from build123d import *

# Parameters (mm, degrees)
SKETCH_1_R          = 29.5
EXTRUDE_1_DEPTH     = 6.6
SKETCH_2_R          = 2
CUT_EXTRUDE_1_DEPTH = 6.6
SKETCH_3_R          = 4
CUT_EXTRUDE_2_DEPTH = 6.6


with BuildPart() as part:
    # 草图1 → 凸台-拉伸1 (new body)
    with BuildSketch(Plane(origin=(0, 0, 0), x_dir=(0, 0, -1), z_dir=(1, 0, 0))):
        Circle(SKETCH_1_R)
    extrude(amount=EXTRUDE_1_DEPTH)

    # 草图2 → 切除-拉伸1 (cut)
    with BuildSketch(Plane(origin=(6.6, 0, 0), x_dir=(0, 0, -1), z_dir=(1, 0, 0))):
        with Locations((0, 17.25)):
            Circle(SKETCH_2_R)
        with Locations((14.938938215, 8.625)):
            Circle(SKETCH_2_R)
        with Locations((14.938938215, -8.625)):
            Circle(SKETCH_2_R)
        with Locations((0, -17.25)):
            Circle(SKETCH_2_R)
        with Locations((-14.938938215, -8.625)):
            Circle(SKETCH_2_R)
        with Locations((-14.938938215, 8.625)):
            Circle(SKETCH_2_R)
    extrude(amount=-CUT_EXTRUDE_1_DEPTH, mode=Mode.SUBTRACT)

    # 草图3 → 切除-拉伸2 (cut)
    with BuildSketch(Plane(origin=(6.6, 0, 0), x_dir=(0, 0, -1), z_dir=(1, 0, 0))):
        Circle(SKETCH_3_R)
    extrude(amount=-CUT_EXTRUDE_2_DEPTH, mode=Mode.SUBTRACT)


solid = part.part
Source: CAD feature listing. Evaluate the final solid. Frame: model axes, mm. Round coordinates to 2 decimals unless told otherwise and drop trailing zeros. Write each loop counter-clockwise with the first axis right and the second up, starting at its lowest first coordinate (ties: lowest second). Pieces come first, ordered by that corner, then holes. Notation, with made-up numbers: M -1,-33 L 3,-33 A14 cw 3,-13 Z; hole C -13,5 d4. An arc over 180 degrees is marked long. One line per item, written item: value. Start each with the question number.
Item 1: Section query C-C (y = -9.5). Return the cut outline in (x, z).
Item 2: Section query A-A (y = 0). Return the cut outline in (x, z).
Item 3: Ray query, L1, parallel to Z at x = 3, y = -7.5; L2, parallel to Z at x = 2.25, y = 8; L3, parallel to Z at x = 4.75, y = -16.5. Return the intervals inside material, ascending. Write a range as from..to.
Item 4: Section query B-B (z = 0). Return the cut outline in (x, y).
Item 5: Pin query (flat end, axial travel): pin 1 (1.5 mm diameter, centred on x = 2, z = -8.5, fed in from +Y); pin 2 (3 mm diameter, centred on y = 17.25, z = 0, fed in from -X); pin 3 (1 mm diameter, centred on x = 4, z = -10, fed in from +Y); pin 4 (3 mm diameter, centred on x = 0.5, z = -8, fed in from +Y) (3 decimals). Return the tip coordinate at first contact, or that it passes through.
Item 6: Section query D-D (x = 3). Return the cut outline in (y, z) (3 decimals), plus the area to 3 significant figures.
Item 7: Mould query, pull axis Y, two halves, no side actions, for faces 1 (the cylindrical face through (3.25, 8.86, -28.14)), 2 (the flat face through (0, -6, 0)), 3 (the cylindrical face through (3.35, 8.71, -12.94)). Classes: pulls with the +Y half, pulls with the -Y half, needs draft (parallel to the pull), parting line crosses it, or undercut.
Result set:
1. outline: M 0,-27.93 L 6.6,-27.93 L 6.6,-16.74 L 0,-16.74 Z; M 0,-13.14 L 6.6,-13.14 L 6.6,13.14 L 0,13.14 Z; M 0,16.74 L 6.6,16.74 L 6.6,27.93 L 0,27.93 Z
2. outline: M 0,-29.5 L 6.6,-29.5 L 6.6,-4 L 0,-4 Z; M 0,4 L 6.6,4 L 6.6,29.5 L 0,29.5 Z
3. L1: z = -28.53..-16.59, -13.29..13.29, 16.59..28.53
3. L2: z = -28.39..-16.84, -13.04..13.04, 16.84..28.39
3. L3: z = -24.45..-1.85, 1.85..24.45
4. outline: M 0,-29.5 L 6.6,-29.5 L 6.6,-19.25 L 0,-19.25 Z; M 0,-15.25 L 6.6,-15.25 L 6.6,-4 L 0,-4 Z; M 0,4 L 6.6,4 L 6.6,15.25 L 0,15.25 Z; M 0,19.25 L 6.6,19.25 L 6.6,29.5 L 0,29.5 Z
5. pin 1: stops at y = 28.46
5. pin 2: passes through
5. pin 3: stops at y = 27.93
5. pin 4: stops at y = 28.775
6. outline: C 0,0 d59; hole C -17.25,0 d4; hole C -8.625,-14.939 d4; hole C -8.625,14.939 d4; hole C 0,0 d8; hole C 8.625,-14.939 d4; hole C 8.625,14.939 d4; hole C 17.25,0 d4
6. area: 2,610 mm²
7. face 1: parting line crosses it
7. face 2: needs draft
7. face 3: undercut
